Geometry: final body of the model. Coordinates: model frame, mm. A direction names the side the tool comes from. Give positions to 0.01 mm unless a question says otherwise; leave off trailing zeros. Loops run counter-clockwise (first coordinate to the right, second up) from the corner with the lowest first, then second, coordinate; pieces in that order, holes last.
from build123d import *

# Parameters (mm, degrees)
SALIENTE_EXTRUIR1_DEPTH = 2
CROQUIS2_R              = 2.05
CORTAR_EXTRUIR1_DEPTH   = 3
CORTAR_EXTRUIR3_REACH   = 4
CORTAR_EXTRUIR4_REACH   = 4
CROQUIS5_W              = 15
CROQUIS5_H              = 2


with BuildPart() as part:
    # Croquis1 → Saliente-Extruir1 (new body)
    with BuildSketch(Plane(origin=(0, 0, 0), x_dir=(1, 0, 0), z_dir=(0, 1, 0))):
        Polygon((94, -40), (50, -40), (50, 50), (-50, 50), (-50, -40), (-94, -40), (-94, -68.768453788), (-74.193903104, -125.32), (74.193903104, -125.32), (94, -68.768453788), align=None)
    extrude(amount=SALIENTE_EXTRUIR1_DEPTH)

    # Croquis2 → Cortar-Extruir1 (cut, through all)
    with BuildSketch(Plane(origin=(0, 2, 0), x_dir=(1, 0, 0), z_dir=(0, 1, 0))):
        with Locations((-45.45, -45.45)):
            Circle(CROQUIS2_R)
        with Locations((45.45, -45.45)):
            Circle(CROQUIS2_R)
        with Locations((-45.45, 45.45)):
            Circle(CROQUIS2_R)
        with Locations((45.45, 45.45)):
            Circle(CROQUIS2_R)
    extrude(amount=-CORTAR_EXTRUIR1_DEPTH, mode=Mode.SUBTRACT)

    # Croquis4 → Cortar-Extruir3 (cut, up to next)
    with BuildSketch(Plane(origin=(0, 2, 0), x_dir=(1, 0, 0), z_dir=(0, 1, 0)), mode=Mode.PRIVATE) as cortar_extruir3_sk1:
        Polygon((50, -68), (64.601532017, -68), (54.332763081, -97.32), (50, -97.32), (50, -115.32), (67.10063881, -115.32), (84, -67.067938511), (84, -50), (50, -50), align=None)
    cortar_extruir3_tool1 = extrude(cortar_extruir3_sk1.sketch, amount=-CORTAR_EXTRUIR3_REACH, mode=Mode.PRIVATE) & part.part
    add(cortar_extruir3_tool1.solids().sort_by_distance((66.115396, 2, 78.737968))[0], mode=Mode.SUBTRACT)

    # Croquis5 → Cortar-Extruir4 (cut, up to next)
    with BuildSketch(Plane(origin=(0, 2, 0), x_dir=(1, 0, 0), z_dir=(0, 1, 0)), mode=Mode.PRIVATE) as cortar_extruir4_sk1:
        with Locations((29.306096896, -51.35767988)):
            Rectangle(CROQUIS5_W, CROQUIS5_H)
    cortar_extruir4_tool1 = extrude(cortar_extruir4_sk1.sketch, amount=-CORTAR_EXTRUIR4_REACH, mode=Mode.PRIVATE) & part.part
    add(cortar_extruir4_tool1.solids().sort_by_distance((29.306097, 2, 51.35768))[0], mode=Mode.SUBTRACT)
    # Croquis5 → Cortar-Extruir4 (cut, up to next)
    with BuildSketch(Plane(origin=(0, 2, 0), x_dir=(1, 0, 0), z_dir=(0, 1, 0)), mode=Mode.PRIVATE) as cortar_extruir4_sk2:
        with Locations((-66.693903104, -51.35767988)):
            Rectangle(CROQUIS5_W, CROQUIS5_H)
    cortar_extruir4_tool2 = extrude(cortar_extruir4_sk2.sketch, amount=-CORTAR_EXTRUIR4_REACH, mode=Mode.PRIVATE) & part.part
    add(cortar_extruir4_tool2.solids().sort_by_distance((-66.693903, 2, 51.35768))[0], mode=Mode.SUBTRACT)
    # Croquis5 → Cortar-Extruir4 (cut, up to next)
    with BuildSketch(Plane(origin=(0, 2, 0), x_dir=(1, 0, 0), z_dir=(0, 1, 0)), mode=Mode.PRIVATE) as cortar_extruir4_sk3:
        with Locations((-36.693903104, -51.35767988)):
            Rectangle(CROQUIS5_W, CROQUIS5_H)
    cortar_extruir4_tool3 = extrude(cortar_extruir4_sk3.sketch, amount=-CORTAR_EXTRUIR4_REACH, mode=Mode.PRIVATE) & part.part
    add(cortar_extruir4_tool3.solids().sort_by_distance((-36.693903, 2, 51.35768))[0], mode=Mode.SUBTRACT)
    # Croquis5 → Cortar-Extruir4 (cut, up to next)
    with BuildSketch(Plane(origin=(0, 2, 0), x_dir=(1, 0, 0), z_dir=(0, 1, 0)), mode=Mode.PRIVATE) as cortar_extruir4_sk4:
        with Locations((-0.693903104, -51.35767988)):
            Rectangle(CROQUIS5_W, CROQUIS5_H)
    cortar_extruir4_tool4 = extrude(cortar_extruir4_sk4.sketch, amount=-CORTAR_EXTRUIR4_REACH, mode=Mode.PRIVATE) & part.part
    add(cortar_extruir4_tool4.solids().sort_by_distance((-0.693903, 2, 51.35768))[0], mode=Mode.SUBTRACT)
    # Croquis5 → Cortar-Extruir4 (cut, up to next)
    with BuildSketch(Plane(origin=(0, 2, 0), x_dir=(1, 0, 0), z_dir=(0, 1, 0)), mode=Mode.PRIVATE) as cortar_extruir4_sk5:
        with Locations((-66.693903104, -111.10767988)):
            Rectangle(CROQUIS5_W, CROQUIS5_H)
    cortar_extruir4_tool5 = extrude(cortar_extruir4_sk5.sketch, amount=-CORTAR_EXTRUIR4_REACH, mode=Mode.PRIVATE) & part.part
    add(cortar_extruir4_tool5.solids().sort_by_distance((-66.693903, 2, 111.10768))[0], mode=Mode.SUBTRACT)
    # Croquis5 → Cortar-Extruir4 (cut, up to next)
    with BuildSketch(Plane(origin=(0, 2, 0), x_dir=(1, 0, 0), z_dir=(0, 1, 0)), mode=Mode.PRIVATE) as cortar_extruir4_sk6:
        with Locations((-36.693903104, -111.10767988)):
            Rectangle(CROQUIS5_W, CROQUIS5_H)
    cortar_extruir4_tool6 = extrude(cortar_extruir4_sk6.sketch, amount=-CORTAR_EXTRUIR4_REACH, mode=Mode.PRIVATE) & part.part
    add(cortar_extruir4_tool6.solids().sort_by_distance((-36.693903, 2, 111.10768))[0], mode=Mode.SUBTRACT)
    # Croquis5 → Cortar-Extruir4 (cut, up to next)
    with BuildSketch(Plane(origin=(0, 2, 0), x_dir=(1, 0, 0), z_dir=(0, 1, 0)), mode=Mode.PRIVATE) as cortar_extruir4_sk7:
        with Locations((-0.693903104, -111.10767988)):
            Rectangle(CROQUIS5_W, CROQUIS5_H)
    cortar_extruir4_tool7 = extrude(cortar_extruir4_sk7.sketch, amount=-CORTAR_EXTRUIR4_REACH, mode=Mode.PRIVATE) & part.part
    add(cortar_extruir4_tool7.solids().sort_by_distance((-0.693903, 2, 111.10768))[0], mode=Mode.SUBTRACT)
    # Croquis5 → Cortar-Extruir4 (cut, up to next)
    with BuildSketch(Plane(origin=(0, 2, 0), x_dir=(1, 0, 0), z_dir=(0, 1, 0)), mode=Mode.PRIVATE) as cortar_extruir4_sk8:
        with Locations((29.306096896, -111.10767988)):
            Rectangle(CROQUIS5_W, CROQUIS5_H)
    cortar_extruir4_tool8 = extrude(cortar_extruir4_sk8.sketch, amount=-CORTAR_EXTRUIR4_REACH, mode=Mode.PRIVATE) & part.part
    add(cortar_extruir4_tool8.solids().sort_by_distance((29.306097, 2, 111.10768))[0], mode=Mode.SUBTRACT)


solid = part.part
Item 1: Section query D-D on z = -12. Return loops of the section in (x, y), plus the area to 3 significant figures.
Values follow:
outline: (-50, 0) - (50, 0) - (50, 2) - (-50, 2) - close
area: 200 mm2
Item 2: Draft query along X for faces 1 (the face through (83.96, 0.99, 97.44)), 2 (the face through (59.54, 1.01, 82.45)), 3 (the face through (-44.504, 1.014, 47.269)), 4 (the face through (-84.236, 0.986, 96.648)). Return one class per face: +X half, -X half, draft (parallel to the pull), parting line (faces both ways), or undercut.
Values follow:
face 1: +X half
face 2: undercut
face 3: undercut
face 4: -X half
Item 3: Section query C-C on y = 0.7. Give the number of separate pieces and of enclosed holes in the cut face, plus the area to 3 significant figures.
Values follow:
separate pieces: 1
enclosed holes: 13
area: 22,100 mm2
Item 4: Section query A-A on x = -36. Return loops of the section in (y, z), plus the area to 3 significant figures.
Values follow:
outline: (0, -50) - (2, -50) - (2, 50.36) - (0, 50.36) - close; (0, 52.36) - (2, 52.36) - (2, 110.11) - (0, 110.11) - close; (0, 112.11) - (2, 112.11) - (2, 125.32) - (0, 125.32) - close
area: 343 mm2
Item 5: Section query B-B on x = 72. Return loops of the section in (y, z), plus the area to 3 significant figures.
Values follow:
outline: (0, 40) - (2, 40) - (2, 50) - (0, 50) - close; (0, 101.33) - (2, 101.33) - (2, 125.32) - (0, 125.32) - close
area: 68.0 mm2
Item 6: Pin query (flat end, axial travel): pin 1 (1 mm diameter, centred on x = 69, y = 1.5, fed in from -Z); pin 2 (1 mm diameter, centred on y = 1.5, z = 111, fed in from -X). Return the tip coordinate at first contact, or that it passes through.
Values follow:
pin 1: stops at z = 40
pin 2: stops at x = -79.38
Item 7: Set-up query: faces 5 (the face through (75.432, 1.014, 91.532)), 6 (the face through (-1, 0, 36)). Return all of +Z, -Z, +X, -X, +Y, -Y with unobstructed straight access to the full face (end or side cutting, diameter ignored); none if empty.
Values follow:
face 5: +Y, -Y
face 6: +Z, -Z, +X, -X, -Y
Item 8: Ray query, probe 1 along X at (y, z) = (1.35, -45.45); probe 2 along Z at (x, y) = (45.45, 1.2); probe 3 along Z at (x, y) = (-36, 0.9). Return the intervals inside material, ascending.
Values follow:
probe 1: x = -50 to -47.5, -43.4 to 43.4, 47.5 to 50
probe 2: z = -50 to -47.5, -43.4 to 43.4, 47.5 to 125.32
probe 3: z = -50 to 50.36, 52.36 to 110.11, 112.11 to 125.32
